Check sheet for the modelled part. Datum: model origin and axes. Units: mm. A direction names the side the tool comes from. Round coordinates to 2 decimals unless told otherwise and drop trailing zeros. Loops run counter-clockwise (first coordinate to the right, second up) from the corner with the lowest first, then second, coordinate; pieces in that order, holes last. Notation, with made-up numbers: (42, 68.5) -> (93, 68.5) arc R15 cw to (93, 89.5) -> close; hole circle Ø2 at (57, -1). An arc over 180 degrees is marked (long way). Return JSON: item names as keys, results as strings.
from build123d import *

# Parameters (mm, degrees)
BOSS_EXTRUDE1_DEPTH = 304.8
SKETCH2_R           = 3.175
BOSS_EXTRUDE2_DEPTH = 17.3228
FILLET1_R           = 1.524
SKETCH3_W           = 6.35
SKETCH3_H           = 1.1684


with BuildPart() as part:
    # Sketch1 → Boss-Extrude1 (new body)
    with BuildSketch(Plane.XY):
        Polygon((-6.35, 3.666174209), (-6.35, -3.666174209), (0, -7.332348419), (6.35, -3.666174209), (6.35, 3.666174209), (0, 7.332348419), align=None)
    extrude(amount=BOSS_EXTRUDE1_DEPTH)

    # Sketch2 → Boss-Extrude2 (add)
    with BuildSketch(Plane.XY.offset(304.8)):
        Circle(SKETCH2_R)
    extrude(amount=BOSS_EXTRUDE2_DEPTH)

    # Fillet1
    fillet1_edges = [part.edges().sort_by_distance(p)[0] for p in [
        (-3.175, 0, 304.8),
    ]]
    fillet(fillet1_edges, radius=FILLET1_R)

    # Sketch3 → Cut-Revolve1 (revolve, cut)
    with BuildSketch(Plane(origin=(0, 0, 0), x_dir=(1, 0, 0), z_dir=(0, 1, 0))):
        with Locations((-8.2042, -295.8338)):
            Rectangle(SKETCH3_W, SKETCH3_H)
    revolve(axis=Axis((0, 0, 330.02530499), (0, 0, -1)), mode=Mode.SUBTRACT)


solid = part.part
Q1. Section check B-B (y = 0). Record the boundary of the cut face in (x, z) (3 decimals), then the cut area to 3 significant figures.
Results list:
{"outline": "(-6.35, 0) -> (6.35, 0) -> (6.35, 295.25) -> (5.029, 295.25) -> (5.029, 296.418) -> (6.35, 296.418) -> (6.35, 304.8) -> (4.699, 304.8) arc R1.524 cw to (3.175, 306.324) -> (3.175, 322.123) -> (-3.175, 322.123) -> (-3.175, 306.324) arc R1.524 cw to (-4.699, 304.8) -> (-6.35, 304.8) -> (-6.35, 296.418) -> (-5.029, 296.418) -> (-5.029, 295.25) -> (-6.35, 295.25) -> close", "area": "3,980 mm^2"}
Q2. Go/stop test with flat-tipped pins: pin 1 (4 mm diameter, centred on y = 6, z = 104.5, fed in from +X); pin 2 (2 mm diameter, centred on x = 4.5, y = 6, fed in from -Z); pin 3 (5 mm diameter, centred on x = 3, z = 127.5, fed in from +Y); pin 4 (2 mm diameter, centred on x = -2.5, z = 160.5, fed in from +Y). Record where each tip stops, or that it passes through.
Results list:
{"pin 1": "x = 5.77", "pin 2": "through", "pin 3": "y = 7.04", "pin 4": "y = 6.47"}
Q3. Material ranges on line 1 (Z direction, x = 1.5, y = 5.5); line 2 (Z direction, x = 3, y = 3.5); line 3 (Y direction, x = 4, z = 230), recorded low to high.
Results list:
{"line 1": "0 to 295.25, 296.42 to 304.8", "line 2": "0 to 304.8", "line 3": "-5.02 to 5.02"}
Q4. Draft check along Z on faces 4 (the flat face through (-3.219, -5.474, 300.55)), 5 (the flat face through (0, 0, 0)), 6 (the flat face through (0, -5.4, 295.25)), 7 (the flat face through (0, -5, 304.8)). Enter one of: released by +Z, released by -Z, zero draft, split by the parting line, or undercut.
Results list:
{"face 4": "zero draft", "face 5": "released by -Z", "face 6": "undercut", "face 7": "released by +Z"}
Q5. Tool access check on faces 1 (the cylindrical face through (-0.69, -3.1, 314.11)), 2 (the flat face through (0, -5.4, 296.418)), 3 (the flat face through (6.35, 0, 146)). Record the directions out of +Z, -Z, +X, -X, +Y, -Y that give a thin tool (end or side, any length) a straight path to the whole face; none if there is none.
Results list:
{"face 1": "+Z", "face 2": "none", "face 3": "+Z, -Z, +X, +Y, -Y"}
Q6. Section check A-A (z = 184.5). Record the boundary of the cut face in (x, y).
Results list:
{"outline": "(-6.35, -3.67) -> (0, -7.33) -> (6.35, -3.67) -> (6.35, 3.67) -> (0, 7.33) -> (-6.35, 3.67) -> close"}
